Verification items for the finished model (mm, model axes). A direction names the side the tool comes from. Coordinates: 2 decimals unless noted, no trailing zeros. Loops run counter-clockwise (first coordinate to the right, second up) from the corner with the lowest first, then second, coordinate; pieces in that order, holes last. Notation, with made-up numbers: M -9,-27 L -5,-27 A23 cw -5,6 Z; hole C 61.5,-28.5 d7. An arc over 180 degrees is marked long. Write item = value, one per line. Start each with the question number.
Autodesk Inventor part; units mm, degrees
ref_plane "Work Plane1" through (0, 0, 0) normal (0, 0, 1) x (1, 0, 0)
ref_plane "YZ Plane" through (0, 0, 0) normal (1, 0, 0) x (0, 1, 0)
ref_plane "XZ Plane" through (0, 0, 0) normal (0, 1, 0) x (-1, 0, 0)
ref_plane "Work Plane1" through (0, 0, 0) normal (0, 0, 1) x (1, 0, 0)
sketch "Sketch1" plane through (0, 0, 0) normal (0, 0, 1) x (1, 0, 0)
  arc A0 (13.19, -29.76) -> (17, -25.95) centre (13.19, -25.95) ccw
  line L0 (17, -25.95) -> (17, -23.57)
  arc A1 (23.57, -17) -> (17, -23.57) centre (23.57, -23.57) ccw
  line L1 (23.57, -17) -> (25.95, -17)
  arc A2 (25.95, -17) -> (29.76, -13.19) centre (25.95, -13.19) ccw
  line L2 (29.76, -13.19) -> (29.76, 13.19)
  arc A3 (29.76, 13.19) -> (25.95, 17) centre (25.95, 13.19) ccw
  line L3 (25.95, 17) -> (23.57, 17)
  arc A4 (17, 23.57) -> (23.57, 17) centre (23.57, 23.57) ccw
  line L4 (17, 23.57) -> (17, 25.95)
  arc A5 (17, 25.95) -> (13.19, 29.76) centre (13.19, 25.95) ccw
  line L5 (13.19, 29.76) -> (-13.19, 29.76)
  arc A6 (-13.19, 29.76) -> (-17, 25.95) centre (-13.19, 25.95) ccw
  line L6 (-17, 25.95) -> (-17, 23.57)
  arc A7 (-23.57, 17) -> (-17, 23.57) centre (-23.57, 23.57) ccw
  line L7 (-23.57, 17) -> (-25.95, 17)
  arc A8 (-25.95, 17) -> (-29.76, 13.19) centre (-25.95, 13.19) ccw
  line L8 (-29.76, 13.19) -> (-29.76, -13.19)
  arc A9 (-29.76, -13.19) -> (-25.95, -17) centre (-25.95, -13.19) ccw
  line L9 (-25.95, -17) -> (-23.57, -17)
  arc A10 (-17, -23.57) -> (-23.57, -17) centre (-23.57, -23.57) ccw
  line L10 (-17, -23.57) -> (-17, -25.95)
  arc A11 (-17, -25.95) -> (-13.19, -29.76) centre (-13.19, -25.95) ccw
  line L11 (-13.19, -29.76) -> (13.19, -29.76)
  line L12 (49.95, 90) -> (49.95, -90)
  arc A12 (13.19, -29.96) -> (17.2, -25.95) centre (13.19, -25.95) ccw
  line L13 (17.2, -25.95) -> (17.2, -23.57)
  arc A13 (23.57, -17.2) -> (17.2, -23.57) centre (23.57, -23.57) ccw
  line L14 (23.57, -17.2) -> (25.95, -17.2)
  arc A14 (25.95, -17.2) -> (29.96, -13.19) centre (25.95, -13.19) ccw
  line L15 (29.96, -13.19) -> (29.96, 13.19)
  arc A15 (29.96, 13.19) -> (25.95, 17.2) centre (25.95, 13.19) ccw
  line L16 (25.95, 17.2) -> (23.57, 17.2)
  arc A16 (17.2, 23.57) -> (23.57, 17.2) centre (23.57, 23.57) ccw
  line L17 (17.2, 23.57) -> (17.2, 25.95)
  arc A17 (17.2, 25.95) -> (13.19, 29.96) centre (13.19, 25.95) ccw
  line L18 (13.19, 29.96) -> (-13.19, 29.96)
  arc A18 (-13.19, 29.96) -> (-17.2, 25.95) centre (-13.19, 25.95) ccw
  line L19 (-17.2, 25.95) -> (-17.2, 23.57)
  arc A19 (-23.57, 17.2) -> (-17.2, 23.57) centre (-23.57, 23.57) ccw
  line L20 (-23.57, 17.2) -> (-25.95, 17.2)
  arc A20 (-25.95, 17.2) -> (-29.96, 13.19) centre (-25.95, 13.19) ccw
  line L21 (-29.96, 13.19) -> (-29.96, -13.19)
  arc A21 (-29.96, -13.19) -> (-25.95, -17.2) centre (-25.95, -13.19) ccw
  line L22 (-25.95, -17.2) -> (-23.57, -17.2)
  arc A22 (-17.2, -23.57) -> (-23.57, -17.2) centre (-23.57, -23.57) ccw
  line L23 (-17.2, -23.57) -> (-17.2, -25.95)
  arc A23 (-17.2, -25.95) -> (-13.19, -29.96) centre (-13.19, -25.95) ccw
  line L24 (-13.19, -29.96) -> (13.19, -29.96)
  line L25 (0, -29.96) -> (0, -34.96)
  line L26 (0, -34.96) -> (49.95, -34.96)
  line L27 (0, 29.96) -> (0, 34.96)
  line L28 (0, 34.96) -> (49.95, 34.96)
  point P0 (0, 0)
  dimension "d0" = 0.2
  dimension "d1" = 5
extrude "Extrusion1" add sketch "Sketch1" along normal blind 10 contours L12 L26 L25 L24 A12 L13 A13 L14 A14 L15 A15 L16 A16 L17 A17 L18 L27 L28
fillet "Fillet1" radius 2 4 edges at (0, -29.96, 5) (0, -34.96, 5) (0, 34.96, 5) (0, 29.96, 5)
sketch "Sketch2" plane through (49.95, -34.96, 0) normal (1, 0, 0) x (0, 0, -1)
  line L0 (-10, 0) -> (-10, 69.92)
  line L1 (0, 0) -> (-10, 0)
  line L2 (0, 69.92) -> (-10, 69.92)
  line L3 (0, 0) -> (0, 69.92)
  point P0 (0, 34.96)
  point P1 (-5, 15)
  point P2 (-5, 54.92)
  point P3 (-5, 69.92)
  dimension "d5" = 15
  dimension "d6" = 15
hole "Hole1" at (49.95, -19.96, 5) at (49.95, 19.96, 5) direction (-1, 0, 0) diameter 3.242 depth 15 tip angle 118
properties part number "nema23steun 10 mm"
Q1. Sectioned sample at A-A on x = 5.5. Record the cut outline in (y, z).
Q2. Sectioned sample at C-C on y = 10. Record the cut outline in (x, z).
Q3. Gauge pin test, flat ends, axial feed: pin 1 (5 mm diameter, centred on y = 19.96, z = 5, fed in from -X); pin 2 (0.7 mm diameter, centred on y = 25, z = 6, fed in from -X); pin 3 (2.5 mm diameter, centred on y = -19.96, z = 5, fed in from +X). Record the tip position at first contact, or that the pin passes through.
Q4. Sectioned sample at B-B on z = 1.5. Record the cut outline in (x, y).
Q5. Mould release check, pull along Z, two halves, no side actions. Record for faces 3 (the face through (34, -20, 5)), 4 (the face through (30.2, 0.5, 0)), 5 (the face through (19.016, -19.116, 4.93)): +Z half, -Z half, draft (parallel to the pull), parting line (faces both ways), or undercut.
Q6. Set-up check for faces 1 (the face through (8, -29.96, 5)), 2 (the face through (34, 20, 5)): record each of +Z, -Z, +X, -X, +Y, -Y from which the full face is reachable in a straight line by a thin tool's end or side.
Q7. Scan lines: L1, parallel to Y at x = 45.75, z = 5; L2, parallel to Z at x = 44, y = -19.96; L3, parallel to Y at x = 23.5, z = 3. Record each from-to range of solid material in increasing order. Write a range as [from, to].
Solutions:
q1.outline = M -34.96,0 L -29.96,0 L -29.96,10 L -34.96,10 Z; M 29.96,0 L 34.96,0 L 34.96,10 L 29.96,10 Z
q2.outline = M 29.96,0 L 49.95,0 L 49.95,10 L 29.96,10 Z
q3.pin_1 = 17.3
q3.pin_2 = 17.2
q3.pin_3 = 34.73
q4.outline = M 0,-32.96 A2 ccw 2,-34.96 L 49.95,-34.96 L 49.95,34.96 L 2,34.96 A2 ccw 0,32.96 L 0,31.96 A2 ccw 2,29.96 L 13.19,29.96 A4.01 cw 17.2,25.95 L 17.2,23.57 A6.37 ccw 23.57,17.2 L 25.95,17.2 A4.01 cw 29.96,13.19 L 29.96,-13.19 A4.01 cw 25.95,-17.2 L 23.57,-17.2 A6.37 ccw 17.2,-23.57 L 17.2,-25.95 A4.01 cw 13.19,-29.96 L 2,-29.96 A2 ccw 0,-31.96 Z
q5.face_3 = undercut
q5.face_4 = -Z half
q5.face_5 = draft
q6.face_1 = +Z, -Z, -X
q6.face_2 = +X
q7.L1 = [-34.96, -21.58], [-18.34, 18.34], [21.58, 34.96]
q7.L2 = [0, 3.38], [6.62, 10]
q7.L3 = [-34.96, -17.2], [17.2, 34.96]
